```python
from build123d import *

# Parameters (mm, degrees)
SKETCH_1_W          = 28
SKETCH_1_H          = 37.9
EXTRUDE_1_DEPTH     = 3
HOLE_WIZARD_M4_1_D  = 3.3
CUT_EXTRUDE_1_DEPTH = 8
FILLET_1_R          = 2
CUT_EXTRUDE_2_DEPTH = 8
FILLET_3_R          = 2
HOLE_WIZARD_M3_1_D  = 2.5


with BuildPart() as part:
    # 草图1 → 凸台-拉伸1 (new, symmetric)
    with BuildSketch(Plane.XY):
        Rectangle(SKETCH_1_W, SKETCH_1_H)
    extrude(amount=EXTRUDE_1_DEPTH, both=True)

    # M4 螺纹孔1 (through all)
    with Locations(Plane.XY.offset(3)):
        with Locations((-10, 14.95), (10, 14.95), (10, -14.95), (-10, -14.95)):
            Hole(HOLE_WIZARD_M4_1_D / 2)

    # 草图5 → 切除-拉伸1 (cut)
    with BuildSketch(Plane.XY.offset(3)):
        with BuildLine():
            ThreePointArc((-10, -10.95), (-7.171572875, -12.121572875), (-6, -14.95))
            Line((-6, -14.95), (6, -14.95))
            ThreePointArc((6, -14.95), (7.171572875, -12.121572875), (10, -10.95))
            Line((10, -10.95), (10, 10.95))
            ThreePointArc((10, 10.95), (7.171572875, 12.121572875), (6, 14.95))
            Line((6, 14.95), (-6, 14.95))
            ThreePointArc((-6, 14.95), (-7.171572875, 12.121572875), (-10, 10.95))
            Line((-10, 10.95), (-10, -10.95))
        make_face()
    extrude(amount=-CUT_EXTRUDE_1_DEPTH, mode=Mode.SUBTRACT)

    # 圆角1
    fillet_1_edges = [part.edges().sort_by_distance(p)[0] for p in [
        (14, -18.95, 0),
        (-14, -18.95, 0),
        (-14, 18.95, 0),
        (14, 18.95, 0),
    ]]
    fillet(fillet_1_edges, radius=FILLET_1_R)

    # 草图6 → 切除-拉伸2 (cut)
    with BuildSketch(Plane.XY.offset(3)):
        with BuildLine():
            Line((-11, 11.077016654), (-11, -11.077016654))
            ThreePointArc((-11, -11.077016654), (-10.50401717, -10.981881215), (-10, -10.95))
            Line((-10, -10.95), (-10, 10.95))
            ThreePointArc((-10, 10.95), (-10.50401717, 10.981881215), (-11, 11.077016654))
        make_face()
        with BuildLine():
            Line((11, 11.077016654), (11, -11.077016654))
            ThreePointArc((11, -11.077016654), (10.50401717, -10.981881215), (10, -10.95))
            Line((10, -10.95), (10, 10.95))
            ThreePointArc((10, 10.95), (10.50401717, 10.981881215), (11, 11.077016654))
        make_face()
    extrude(amount=-CUT_EXTRUDE_2_DEPTH, mode=Mode.SUBTRACT)

    # 圆角3
    fillet_3_edges = [part.edges().sort_by_distance(p)[0] for p in [
        (-11, 11.077016654, 0),
        (-11, -11.077016654, 0),
        (11, 11.077016654, 0),
        (11, -11.077016654, 0),
        (6, -14.95, 0),
        (-6, -14.95, 0),
        (-6, 14.95, 0),
        (6, 14.95, 0),
    ]]
    fillet(fillet_3_edges, radius=FILLET_3_R)

    # M3 螺纹孔1 (through all)
    with Locations(Plane(origin=(0, 18.95, 0), x_dir=(1, 0, 0), z_dir=(0, 1, 0))):
        with Locations((0, 0)):
            Hole(HOLE_WIZARD_M3_1_D / 2)


solid = part.part
```
Source: CAD feature listing. Evaluate the final solid. Frame: model axes, mm. A direction names the side the tool comes from. Round coordinates to 2 decimals unless told otherwise and drop trailing zeros. Order: outer loops, then holes, each group sorted by start corner. A loop starts at its lowest first (then second) coordinate and runs counter-clockwise, first axis right, second up. Notation, with made-up numbers: (9.5, -38.75) -> (13.5, -38.75) arc R20 cw to (13.5, -28.75) -> close; hole circle Ø9 at (-22.5, -33.5). An arc over 180 degrees is marked (long way). One line per item, written item: value. Start each with the question number.
Q1. Draft query along Z for faces 1 (the cylindrical face through (0.27, 16.92, 1.22)), 2 (the flat face through (-13, 0, -3)), 3 (the cylindrical face through (13.4, -18.38, 0.04)). Return one class per face: pulls with the +Z half, pulls with the -Z half, needs draft (parallel to the pull), parting line crosses it, or undercut.
Q2. Section query C-C (y = 4.5). Return the cut outline in (x, z), plus the area to 3 significant figures.
Q3. Material intervals for probe 1 along X at (y, z) = (4, 1.5); probe 2 along Y at (x, z) = (-3.5, 2.75); probe 3 along Y at (x, z) = (10, 1.05), sorted ascending.
Q4. Section query A-A (x = 3). Return the cut outline in (y, z), plus the area to 3 significant figures.
Q5. Section query B-B (x = 0). Return the cut outline in (y, z).
Q6. Access query for faces 4 (the cylindrical face through (13.4, 18.38, -0.04)), 5 (the cylindrical face through (7.45, 11.87, 0.04)). Directions: +Z, -Z, +X, -X, +Y, -Y. A direction counts if a zero-diameter tool reaches every point of the face in a straight line with its end or side. Return the directions, or none.
Q7. Section query D-D (y = -16). Return the cut outline in (x, z), plus the area to 3 significant figures.
Q8. Pin query (flat end, axial travel): pin 1 (3 mm diameter, centred on x = -10, y = -14.95, fed in from +Z). Return the tip coordinate at first contact, or that it passes through.
Findings below:
1. face 1: undercut
1. face 2: pulls with the -Z half
1. face 3: needs draft
2. outline: (-14, -3) -> (-11, -3) -> (-11, 3) -> (-14, 3) -> close; (11, -3) -> (14, -3) -> (14, 3) -> (11, 3) -> close
2. area: 36.0 mm²
3. probe 1: -14 to -11, 11 to 14
3. probe 2: -18.95 to -14.95, 14.95 to 18.95
3. probe 3: -18.95 to -16.6, -13.3 to -10.77, 10.77 to 13.3, 16.6 to 18.95
4. outline: (-18.95, -3) -> (-14.95, -3) -> (-14.95, 3) -> (-18.95, 3) -> close; (14.95, -3) -> (18.95, -3) -> (18.95, 3) -> (14.95, 3) -> close
4. area: 48.0 mm²
5. outline: (-18.95, -3) -> (-14.95, -3) -> (-14.95, -1.25) -> (-18.95, -1.25) -> close; (-18.95, 1.25) -> (-14.95, 1.25) -> (-14.95, 3) -> (-18.95, 3) -> close; (14.95, -3) -> (18.95, -3) -> (18.95, -1.25) -> (14.95, -1.25) -> close; (14.95, 1.25) -> (18.95, 1.25) -> (18.95, 3) -> (14.95, 3) -> close
6. face 4: +Z, -Z, +X, +Y
6. face 5: +Z, -Z
7. outline: (-14, -3) -> (-11.27, -3) -> (-11.27, 3) -> (-14, 3) -> close; (-8.73, -3) -> (8.73, -3) -> (8.73, 3) -> (-8.73, 3) -> close; (11.27, -3) -> (14, -3) -> (14, 3) -> (11.27, 3) -> close; hole circle Ø2.5 at (0, 0)
7. area: 133 mm²
8. pin 1: through
